from build123d import *

# Parameters (mm, degrees)
BOSS_EXTRUDE1_DEPTH = 100
CUT_EXTRUDE1_DEPTH  = 8
CUT_EXTRUDE2_DEPTH  = 3
BOSS_EXTRUDE4_DEPTH = 20


with BuildPart() as part:
    # Sketch1 → Boss-Extrude1 (new body)
    with BuildSketch(Plane.XY):
        with BuildLine():
            Line((-20, 0), (-16, 0))
            Line((-16, 0), (-10, 0))
            Line((-10, 0), (0, 0))
            Line((0, 0), (10, 0))
            Line((10, 0), (16, 0))
            Line((16, 0), (20, 0))
            ThreePointArc((20, 0), (0, -20), (-20, 0))
        make_face()
    extrude(amount=BOSS_EXTRUDE1_DEPTH)

    # Sketch2 → Cut-Extrude1 (cut)
    with BuildSketch(Plane(origin=(0, 0, 0), x_dir=(-1, 0, 0), z_dir=(0, 0, -1))):
        with BuildLine():
            Line((-10, 0), (-16, 0))
            ThreePointArc((-16, 0), (0, -16), (16, 0))
            Line((16, 0), (10, 0))
            ThreePointArc((10, 0), (0, -10), (-10, 0))
        make_face()
    extrude(amount=-CUT_EXTRUDE1_DEPTH, mode=Mode.SUBTRACT)

    # Sketch3 → Cut-Extrude2 (cut)
    with BuildSketch(Plane(origin=(0, 0, 0), x_dir=(1, 0, 0), z_dir=(0, 1, 0))):
        with BuildLine():
            Line((5, -25), (5, -60))
            ThreePointArc((5, -60), (0, -65), (-5, -60))
            Line((-5, -60), (-5, -25))
            ThreePointArc((-5, -25), (0, -20), (5, -25))
        make_face()
    extrude(amount=-CUT_EXTRUDE2_DEPTH, mode=Mode.SUBTRACT)

    # Sketch4 → Boss-Extrude4 (add)
    with BuildSketch(Plane.XY.offset(100)):
        with BuildLine():
            Line((-20, 0), (-16, 0))
            ThreePointArc((-16, 0), (0, 16), (16, 0))
            Line((16, 0), (20, 0))
            ThreePointArc((20, 0), (0, 20), (-20, 0))
        make_face()
    extrude(amount=-BOSS_EXTRUDE4_DEPTH)


solid = part.part
Could you check a few things on this model? Use its own coordinates, in mm. A direction names the side the tool comes from. Give positions to 0.01 mm unless a question says otherwise; leave off trailing zeros. Write each loop counter-clockwise with the first axis right and the second up, starting at its lowest first coordinate (ties: lowest second). Pieces come first, ordered by that corner, then holes. Notation, with made-up numbers: (50.5, -32.75) -> (90.5, -32.75) arc R16 ccw to (90.5, -28.75) -> close; hole circle Ø8 at (-12, 84.5). An arc over 180 degrees is marked (long way). Answer as CSV lines item,"result". Start each with the question number.
(1) If we mould it in two halves opening along Y, with no side actions, what happens to faces 5 (the face through (0, -10, 4)), 6 (the face through (-2.6, -19.83, 60.41)), 7 (the face through (5, -1, 42))? For each: +Y half, -Y half, draft (parallel to the pull), parting line (faces both ways), or undercut.
(2) Which directions (+Z, -Z, +X, -X, +Y, -Y) give clear straight access to the entire face, cutting with the end or side of a thin tool? Please do faces 1 (the face through (0, 16, 90)), 2 (the face through (0, -16, 4)), 3 (the face through (3, 16, 80)), 4 (the face through (0, -1, 20)).
(3) If we section it at B-B, the plane z = 6: Write out the boundary of the cut face in (x, y).
(4) Please list where these lines run through material, in increasing order: line 1 (X direction, y = 5, z = 86); line 2 (X direction, y = -0.5, z = 51); line 3 (Z direction, x = -11.5, y = -8).
(5) I'm going to push flat-ended pins straight in: pin 1 Ø2.5 at (y, z) = (-2, 47) entering from +X; pin 2 Ø2 at (y, z) = (-11.5, 29.5) entering from +X; pin 3 Ø1.5 at (x, z) = (13, 74) entering from +Y. Where does each tip first touch, or does it pass through?
(6) If we section it at D-D, the plane z = 92.5: Write out the boundary of the cut face in (x, y).
(7) If we section it at C-C, the plane y = -14.5: Write out the boundary of the cut face in (x, z), and give its area (3 significant figures).
(8) If we section it at A-A, the plane x = 0: Write out the boundary of the cut face in (y, z), and give its area (3 significant figures).
Answer list:
1,face 5,"undercut"
1,face 6,"parting line"
1,face 7,"draft"
2,face 1,"+Z, -Z"
2,face 2,"-Z"
2,face 3,"-Z, +X, -X, +Y"
2,face 4,"+Y"
3,outline,"(-20, 0) arc R20 ccw to (20, 0) -> (16, 0) arc R16 cw to (-16, 0) -> close; (-10, 0) arc R10 ccw to (10, 0) -> close"
4,line 1,"-19.36 to -15.2, 15.2 to 19.36"
4,line 2,"-19.99 to -5, 5 to 19.99"
4,line 3,"8 to 100"
5,pin 1,"x = 19.99"
5,pin 2,"x = 17.02"
5,pin 3,"y = 0"
6,outline,"circle Ø40 at (0, 0); hole (-16, 0) -> (16, 0) arc R16 ccw to start"
7,outline,"(-13.77, 0) -> (-6.76, 0) -> (-6.76, 8) -> (6.76, 8) -> (6.76, 0) -> (13.77, 0) -> (13.77, 100) -> (-13.77, 100) -> close"
7,area,"2,650 mm^2"
8,outline,"(-20, 0) -> (-16, 0) -> (-16, 8) -> (-10, 8) -> (-10, 0) -> (0, 0) -> (0, 20) -> (-3, 20) -> (-3, 65) -> (0, 65) -> (0, 100) -> (-20, 100) -> close; (16, 80) -> (20, 80) -> (20, 100) -> (16, 100) -> close"
8,area,"1,900 mm^2"
